from build123d import *

# Parameters (mm, degrees)
BOSS_EXTRUDE1_DEPTH = 250
SKETCH3_W           = 80
SKETCH3_H           = 90
BOSS_EXTRUDE3_DEPTH = 250
CUT_EXTRUDE1_DEPTH  = 500
CUT_EXTRUDE2_DEPTH  = 500
BOSS_EXTRUDE4_DEPTH = 75
SKETCH7_R           = 82
BOSS_EXTRUDE5_DEPTH = 75
SKETCH8_R           = 86.820358575
BOSS_EXTRUDE6_DEPTH = 90
BOSS_EXTRUDE7_START = 7.5
SKETCH9_R           = 82
BOSS_EXTRUDE7_DEPTH = 7.5
SKETCH10_R          = 86.820358575
BOSS_EXTRUDE8_DEPTH = 7.5
BOSS_EXTRUDE9_DEPTH = 280


with BuildPart() as part:
    # Sketch2 → Boss-Extrude1 (new body)
    with BuildSketch(Plane.XY):
        Polygon((0, 0), (0, 350), (171.438035453, 445), (421.438035453, 445), (421.438035453, 370), (134.808708212, 370), (134.808708212, 90), (360, 90), (360, 0), align=None)
    extrude(amount=-BOSS_EXTRUDE1_DEPTH)

    # Sketch3 → Boss-Extrude3 (add)
    with BuildSketch(Plane.XY):
        with Locations((400, 45)):
            Rectangle(SKETCH3_W, SKETCH3_H)
    extrude(amount=-BOSS_EXTRUDE3_DEPTH)

    # Sketch4 → Cut-Extrude1 (cut)
    with BuildSketch(Plane(origin=(0, 445, 0), x_dir=(1, 0, 0), z_dir=(0, 1, 0))):
        Polygon((171.438035453, 250), (421.438035453, 173.567329635), (421.438035453, 250), align=None)
    extrude(amount=-CUT_EXTRUDE1_DEPTH, mode=Mode.SUBTRACT)

    # Sketch5 → Cut-Extrude2 (cut)
    with BuildSketch(Plane(origin=(0, 90, 0), x_dir=(1, 0, 0), z_dir=(0, 1, 0))):
        Polygon((171.438035453, 250), (529.292603831, 140.837226457), (529.292603831, 329.490615835), align=None)
    extrude(amount=-CUT_EXTRUDE2_DEPTH, mode=Mode.SUBTRACT)

    # Sketch6 → Boss-Extrude4 (add)
    with BuildSketch(Plane(origin=(0, 445, 0), x_dir=(1, 0, 0), z_dir=(0, 1, 0))):
        Polygon((458.366845574, 162.410857278), (421.438035453, 173.567329635), (419.282590182, 0), (458.366845574, 0), align=None)
    extrude(amount=-BOSS_EXTRUDE4_DEPTH)

    # Sketch7 → Boss-Extrude5 (add)
    with BuildSketch(Plane(origin=(0, 445, 0), x_dir=(1, 0, 0), z_dir=(0, 1, 0))):
        with Locations((458.366845574, 81.205428639)):
            Circle(SKETCH7_R)
    extrude(amount=-BOSS_EXTRUDE5_DEPTH)

    # Sketch8 → Boss-Extrude6 (add)
    with BuildSketch(Plane(origin=(0, 90, 0), x_dir=(1, 0, 0), z_dir=(0, 1, 0))):
        with Locations((440, 84.037872492)):
            Circle(SKETCH8_R)
    extrude(amount=-BOSS_EXTRUDE6_DEPTH)

    # Sketch9 → Boss-Extrude7 (add)
    with BuildSketch(Plane(origin=(0, 445, 0), x_dir=(1, 0, 0), z_dir=(0, 1, 0)).offset(BOSS_EXTRUDE7_START)):
        with Locations(Location((458.366845574, 81.205428639, 0), (0, 0, 270))):
            Circle(SKETCH9_R)
    extrude(amount=-BOSS_EXTRUDE7_DEPTH)

    # Sketch10 → Boss-Extrude8 (add)
    with BuildSketch(Plane.XZ):
        with Locations(Location((440, -84.037872492, 0), (0, 0, 104.544878668))):
            Circle(SKETCH10_R)
    extrude(amount=BOSS_EXTRUDE8_DEPTH)

    # Sketch11 → Boss-Extrude9 (add)
    with BuildSketch(Plane(origin=(0, 90, 0), x_dir=(1, 0, 0), z_dir=(0, 1, 0))):
        Polygon((134.808708212, 0), (187.780197763, 42.295296089), (187.780197763, 197.600080779), (134.808708212, 250), align=None)
    extrude(amount=BOSS_EXTRUDE9_DEPTH)


solid = part.part
Work out the finished part from the listing and answer in its coordinate system (mm). A direction names the side the tool comes from. Round coordinates to 2 decimals unless told otherwise and drop trailing zeros. Write each loop counter-clockwise with the first axis right and the second up, starting at its lowest first coordinate (ties: lowest second). Pieces come first, ordered by that corner, then holes.
1) Given pin 1 Ø12 at (x, y) = (189.5, 118.5) entering from +Z; pin 2 Ø4 at (y, z) = (296.5, -98) entering from +X; pin 3 Ø4 at (x, z) = (248, -114) entering from -Y, each flat-ended and moving along its own axis, determine where each tip first touches the part or whether it passes through.
2) A cutting plane is placed at D-D (x = 327). Give the vertices of the cut face in (y, z).
3) A cutting plane is placed at C-C (z = -29.5). Give the vertices of the cut face in (x, y).
4) The mould has two halves that part along Y. Classify faces 4 (the flat face through (439, -7.5, -86)), 5 (the flat face through (328, 90, -97)), 6 (the flat face through (294.69, 408.02, -212.32)): pulls with the +Y half, pulls with the -Y half, needs draft (parallel to the pull), parting line crosses it, or undercut.
5) A cutting plane is placed at A-A (x = 210). Give the vertices of the cut face in (y, z).
6) A cutting plane is placed at B-B (y = 325.5). Give the vertices of the cut face in (x, z), plus the area to 3 significant figures.
7) A tool of negligible diameter and unlimited length cuts with its end or side. For faces 1 (the flat face through (438.892, 408.025, -168.294)), 2 (the flat face through (187.78, 228, -119)), 3 (the flat face through (161.7, 228, -223.4)), from which of +Z, -Z, +X, -X, +Y, -Y can it reach the whole face along a straight path? Write none if from no direction.
8) Straight lines are drawn through the part: line 1 (Y direction, x = 380, z = -157.5); line 2 (X direction, y = 146, z = -128); line 3 (Y direction, x = 367.5, z = -38.5). For each, find the intervals that lie inside material, in ascending order.
Completed:
1. pin 1: stops at z = -38.88
1. pin 2: stops at x = 187.78
1. pin 3: stops at y = 0
2. outline: (0, -202.44) - (90, -202.44) - (90, 0) - (0, 0) - close; (370, -202.44) - (445, -202.44) - (445, 0) - (370, 0) - close
3. outline: (0, 0) - (372.45, 0) - (372.45, -7.5) - (507.55, -7.5) - (507.55, 90) - (171.76, 90) - (171.76, 370) - (522.01, 370) - (522.01, 452.5) - (394.72, 452.5) - (394.72, 445) - (171.44, 445) - (0, 350) - close
4. face 4: pulls with the -Y half
4. face 5: undercut
4. face 6: needs draft
5. outline: (0, -238.21) - (90, -238.21) - (90, 0) - (0, 0) - close; (370, -238.21) - (445, -238.21) - (445, 0) - (370, 0) - close
6. outline: (0, -250) - (134.81, -250) - (187.78, -197.6) - (187.78, -42.3) - (134.81, 0) - (0, 0) - close
6. area: 44,400 mm2
7. face 1: -Z, +X, +Y
7. face 2: +Z, -Z, +X
7. face 3: -Z, +X
8. line 1: y = 0 to 90, 370 to 445
8. line 2: x = 0 to 187.78
8. line 3: y = -7.5 to 90, 370 to 445
